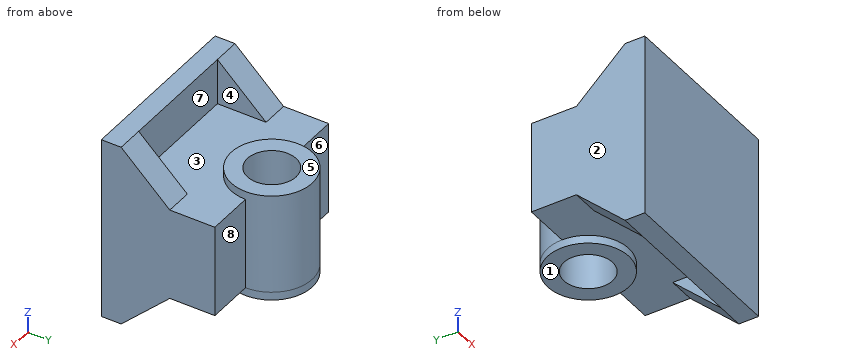
from build123d import *

# Parameters (mm, degrees)
BOSS_EXTRUDE1_DEPTH = 65
BOSS_EXTRUDE2_DEPTH = 10
BOSS_EXTRUDE3_DEPTH = 10
BOSS_EXTRUDE4_DEPTH = 10
BOSS_EXTRUDE5_DEPTH = 10
SKETCH6_R           = 15
BOSS_EXTRUDE6_DEPTH = 34
BOSS_EXTRUDE7_START = 3
SKETCH7_R           = 15
BOSS_EXTRUDE7_DEPTH = 3
SKETCH8_R           = 15
BOSS_EXTRUDE8_DEPTH = 3
CUT_EXTRUDE1_REACH  = 98.743
SKETCH9_R           = 9


with BuildPart() as part:
    # Sketch1 → Boss-Extrude1 (new body)
    with BuildSketch(Plane(origin=(0, 0, 0), x_dir=(0, 0, -1), z_dir=(1, 0, 0))):
        Polygon((-50.255892256, -9.902356902), (-50.255892256, -2.575757576), (-33.255892256, -2.575757576), (-33.255892256, 32.097643098), (0.744107744, 32.097643098), (0.744107744, -2.575757576), (17.744107744, -2.575757576), (17.744107744, -9.902356902), align=None)
    extrude(amount=-BOSS_EXTRUDE1_DEPTH)

    # Sketch2 → Boss-Extrude2 (add)
    with BuildSketch(Plane(origin=(0, 0, 0), x_dir=(0, 0, -1), z_dir=(1, 0, 0))):
        Polygon((-33.255892256, 15.424242424), (-50.255892256, -2.575757576), (-33.255892256, -2.575757576), align=None)
    extrude(amount=-BOSS_EXTRUDE2_DEPTH)

    # Sketch3 → Boss-Extrude3 (add)
    with BuildSketch(Plane.ZY.offset(65)):
        Polygon((33.255892256, 15.424242424), (50.255892256, -2.575757576), (33.255892256, -2.575757576), align=None)
    extrude(amount=-BOSS_EXTRUDE3_DEPTH)

    # Sketch4 → Boss-Extrude4 (add)
    with BuildSketch(Plane.ZY.offset(65)):
        Polygon((-17.744107744, -2.575757576), (-0.744107744, 15.424242424), (-0.744107744, -2.575757576), align=None)
    extrude(amount=-BOSS_EXTRUDE4_DEPTH)

    # Sketch5 → Boss-Extrude5 (add)
    with BuildSketch(Plane(origin=(0, 0, 0), x_dir=(0, 0, -1), z_dir=(1, 0, 0))):
        Polygon((0.744107744, 15.424242424), (17.744107744, -2.575757576), (0.744107744, -2.575757576), align=None)
    extrude(amount=-BOSS_EXTRUDE5_DEPTH)

    # Sketch6 → Boss-Extrude6 (add)
    with BuildSketch(Plane.XY.offset(33.255892256)):
        with Locations((-32.5, 32.097643098)):
            Circle(SKETCH6_R)
    extrude(amount=-BOSS_EXTRUDE6_DEPTH)

    # Sketch7 → Boss-Extrude7 (add)
    with BuildSketch(Plane.XY.offset(33.255892256).offset(BOSS_EXTRUDE7_START)):
        with Locations((-32.5, 32.097643098)):
            Circle(SKETCH7_R)
    extrude(amount=-BOSS_EXTRUDE7_DEPTH)

    # Sketch8 → Boss-Extrude8 (add)
    with BuildSketch(Plane(origin=(0, 0, -0.744107744), x_dir=(-1, 0, 0), z_dir=(0, 0, -1))):
        with Locations(Location((32.5, 32.097643098, 0), (0, 0, 180))):
            Circle(SKETCH8_R)
    extrude(amount=BOSS_EXTRUDE8_DEPTH)

    # Sketch9 → Cut-Extrude1 (cut, up to next)
    with BuildSketch(Plane(origin=(0, 0, -3.744107744), x_dir=(-1, 0, 0), z_dir=(0, 0, -1)), mode=Mode.PRIVATE) as cut_extrude1_sk1:
        with Locations(Location((32.5, 32.097643098, 0), (0, 0, 90))):
            Circle(SKETCH9_R)
    cut_extrude1_tool1 = extrude(cut_extrude1_sk1.sketch, amount=-CUT_EXTRUDE1_REACH, mode=Mode.PRIVATE) & part.part
    add(cut_extrude1_tool1.solids().sort_by_distance((-32.5, 32.097643, -3.744108))[0], mode=Mode.SUBTRACT)


solid = part.part
Geometry check sheet. Reference: the model listing, model coordinates, mm. Face numbers are marked on the shaded views. A direction names the side the tool comes from. Round coordinates to 2 decimals unless told otherwise and drop trailing zeros. Order: outer loops, then holes, each group sorted by start corner. A loop starts at its lowest first (then second) coordinate and runs counter-clockwise, first axis right, second up. Notation, with made-up numbers: M 89,-29.75 L 127,-29.75 A18 cw 127,-19.75 Z; hole C 77.25,10.25 d6. An arc over 180 degrees is marked long. Answer in a Markdown table with one row per item.
(1) Go/stop test with flat-tipped pins: P1, Ø19, axis at x = -59, z = 19, coming from the +Y side; P2, Ø8, axis at x = -29.5, y = 18, coming from the -Z side; P3, Ø1.5, axis at x = -43, y = 4.5, coming from the +Z side. Record where each tip stops, or that it passes through.
Responses:
| item | result |
|---|---|
| P1 | stops at y = 32.1 |
| P2 | stops at z = -3.74 |
| P3 | stops at z = 33.26 |
(2) Draft check along X on the marked faces 1, 2 and 3. Enter one of: released by +X, released by -X, zero draft, split by the parting line, or undercut.
Responses:
| item | result |
|---|---|
| face 1 | zero draft |
| face 2 | released by -X |
| face 3 | undercut |
(3) Scan lines: probe 1 along Y at (x, z) = (-32, 10); probe 2 along Z at (x, y) = (-14, 1); probe 3 along X at (y, z) = (38, 31). Record each from-to range of solid material in increasing order. Write a range as from..to.
Responses:
| item | result |
|---|---|
| probe 1 | y = -9.9..23.11, 41.08..47.09 |
| probe 2 | z = -0.74..33.26 |
| probe 3 | x = -46.29..-39.29, -25.71..-18.71 |
(4) Sectioned sample at C-C, the plane y = 28. Record the cut outline in (x, z), and give its area (3 significant figures).
Responses:
| item | result |
|---|---|
| outline | M -65,-0.74 L -46.93,-0.74 L -46.93,-3.74 L -40.51,-3.74 L -40.51,36.26 L -46.93,36.26 L -46.93,33.26 L -65,33.26 Z; M -24.49,-3.74 L -18.07,-3.74 L -18.07,-0.74 L 0,-0.74 L 0,33.26 L -18.07,33.26 L -18.07,36.26 L -24.49,36.26 Z |
| area | 1,740 mm² |
(5) Sectioned sample at A-A, the plane x = -32.5. Record the cut outline in (y, z).
Responses:
| item | result |
|---|---|
| outline | M -9.9,-17.74 L -2.58,-17.74 L -2.58,-0.74 L 17.1,-0.74 L 17.1,-3.74 L 23.1,-3.74 L 23.1,36.26 L 17.1,36.26 L 17.1,33.26 L -2.58,33.26 L -2.58,50.26 L -9.9,50.26 Z; M 41.1,-3.74 L 47.1,-3.74 L 47.1,36.26 L 41.1,36.26 Z |
(6) Sectioned sample at B-B, the plane z = 35. Record the cut outline in (x, y), and give its area (3 significant figures).
Responses:
| item | result |
|---|---|
| outline | M -65,-9.9 L 0,-9.9 L 0,13.58 L -10,13.58 L -10,-2.58 L -55,-2.58 L -55,13.58 L -65,13.58 Z; C -32.5,32.1 d30; hole C -32.5,32.1 d18 |
| area | 1,250 mm² |
(7) Sectioned sample at D-D, the plane z = 25.5. Record the cut outline in (x, y).
Responses:
| item | result |
|---|---|
| outline | M -65,-9.9 L 0,-9.9 L 0,32.1 L -17.5,32.1 A15 ccw -47.5,32.1 L -65,32.1 Z; hole C -32.5,32.1 d18 |
(8) Tool access check on the marked faces 4, 5, 6, 7 and 8. Record the directions out of +Z, -Z, +X, -X, +Y, -Y that give a thin tool (end or side, any length) a straight path to the whole face; none if there is none.
Responses:
| item | result |
|---|---|
| face 4 | +Z, +Y |
| face 5 | +Z, +X, -X, +Y |
| face 6 | +Z, -Z, -X, +Y |
| face 7 | +Z |
| face 8 | +Z, -Z, +X, +Y |
